Build history of the part. All positions in model axes, mm. Face numbers are marked on the shaded views. A direction names the side the tool comes from. Round coordinates to 2 decimals unless told otherwise and drop trailing zeros. Loops run counter-clockwise (first coordinate to the right, second up) from the corner with the lowest first, then second, coordinate; pieces in that order, holes last. Notation, with made-up numbers: (-8.5, 44.25) - (1.5, 44.25) arc R32 cw to (1.5, 81.25) - close; hole circle Ø5 at (-33.75, 37). An arc over 180 degrees is marked (long way). Put each result on its own line as item: value. Start each with the question number.
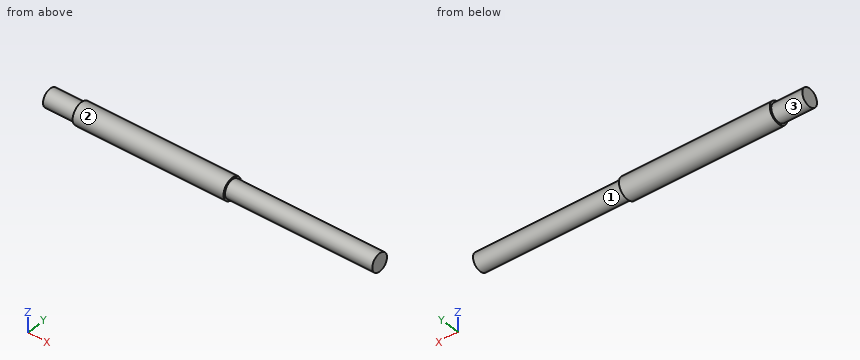
from build123d import *

# Parameters (mm, degrees)
ESQUISSE2_W             = 185.5
ESQUISSE2_H             = 6
ESQUISSE3_R             = 6
ESQUISSE3_R_2           = 5
ENL_V_MAT_EXTRU_1_DEPTH = 83
ENL_V_START             = -17.5
ENL_V_MAT_EXTRU_2_DEPTH = 17.5


with BuildPart() as part:
    # Esquisse2 → Révolution2 (revolve)
    with BuildSketch(Plane(origin=(0, 0, 0), x_dir=(1, 0, 0), z_dir=(0, 1, 0))):
        with Locations((92.75, 3)):
            Rectangle(ESQUISSE2_W, ESQUISSE2_H)
    revolve(axis=Axis((0, 0, -6), (1, 0, 0)))

    # Esquisse3 → Enlèv. mat.-Extru.1 (cut)
    with BuildSketch(Plane(origin=(185.5, 0, 0), x_dir=(0, 0, -1), z_dir=(1, 0, 0))):
        with Locations(Location((6, 0, 0), (0, 0, 180))):
            Circle(ESQUISSE3_R)
        with Locations((6, 0)):
            Circle(ESQUISSE3_R_2, mode=Mode.SUBTRACT)
    extrude(amount=-ENL_V_MAT_EXTRU_1_DEPTH, mode=Mode.SUBTRACT)

    # Esquisse5 → Enlèv. mat.-Extru.2 (cut)
    with BuildSketch(Plane.ZY.offset(ENL_V_START)):
        with BuildLine():
            ThreePointArc((-11, 0), (-6, 5), (-1, 0))
            Line((-1, 0), (0, 0))
            ThreePointArc((0, 0), (-6, 6), (-12, 0))
            Line((-12, 0), (-11, 0))
        make_face()
        with BuildLine():
            Line((0, 0), (-1, 0))
            ThreePointArc((-1, 0), (-6, -5), (-11, 0))
            Line((-11, 0), (-12, 0))
            ThreePointArc((-12, 0), (-6, -6), (0, 0))
        make_face()
    extrude(amount=ENL_V_MAT_EXTRU_2_DEPTH, mode=Mode.SUBTRACT)


solid = part.part
Item 1: Which spindle directions (+Z, -Z, +X, -X, +Y, -Y) get a long thin tool onto all of the face, cutting with end or side? Do the marked faces 1, 2 and 3. Say none if no direction does.
Item 2: Slice it at B-B (y = 0). Give the cut face in (x, z).
Item 3: Slice it at C-C (x = 12). Give the cut face in (y, z).
Item 4: Slice it at D-D (x = 39). Give the cut face in (y, z), plus the area to 3 significant figures.
Item 5: Slice it at A-A (z = -6). Give the cut face in (x, y).
Item 6: Drop flat-ended pins along their axis: pin 1 Ø2 at (x, z) = (87.5, -1) entering from +Y; pin 2 Ø1 at (x, y) = (117.5, 2.5) entering from +Z; pin 3 Ø1 at (x, z) = (118, -7) entering from +Y. Give the stop position or say it passes through.
Item 7: Drill centre lines: probe 1 along Z at (x, y) = (85, 0.5); probe 2 along Z at (x, y) = (163.5, 0.5); probe 3 along X at (y, z) = (4.5, -8.5). Where is each one in solid material? Low to high. Write a range as [from, to].
Computed values:
1. face 1: +X
1. face 2: +X, -X
1. face 3: -X
2. outline: (0, -11) - (17.5, -11) - (17.5, -12) - (102.5, -12) - (102.5, -11) - (185.5, -11) - (185.5, -1) - (102.5, -1) - (102.5, 0) - (17.5, 0) - (17.5, -1) - (0, -1) - close
3. outline: circle Ø10 at (0, -6)
4. outline: circle Ø12 at (0, -6)
4. area: 113 mm^2
5. outline: (0, -5) - (17.5, -5) - (17.5, -6) - (102.5, -6) - (102.5, -5) - (185.5, -5) - (185.5, 5) - (102.5, 5) - (102.5, 6) - (17.5, 6) - (17.5, 5) - (0, 5) - close
6. pin 1: stops at y = 4.47
6. pin 2: stops at z = -1.42
6. pin 3: stops at y = 4.97
7. probe 1: z = [-11.98, -0.02]
7. probe 2: z = [-10.97, -1.03]
7. probe 3: x = [17.5, 102.5]
